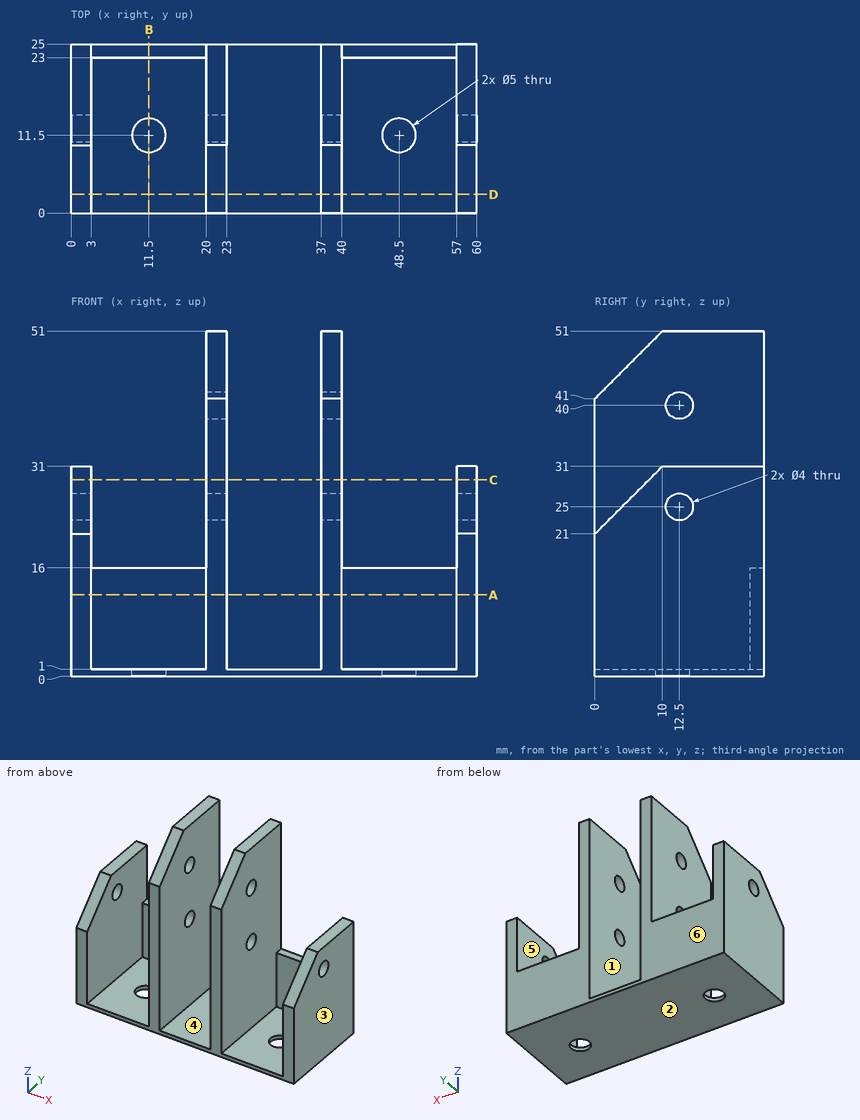
Could you check a few things on this drawing? It's one solid part, dimensions in mm from its lowest x, y, z. A direction names the side the tool comes from. Give positions to 0.01 mm unless a question says otherwise; leave off trailing zeros. Loops run counter-clockwise (first coordinate to the right, second up) from the corner with the lowest first, then second, coordinate; pieces in that order, holes last. Notation, with made-up numbers: (64, 36) -> (102, 36) arc R30 cw to (102, 59) -> close; hole circle Ø7 at (88.5, 17). An arc over 180 degrees is marked (long way). Answer as CSV lines item,"result". Start each with the question number.
(1) We'd pull the mould along X, two halves only. Please class the marked faces 1, 2 and 3: released by +X, released by -X, zero draft, split by the parting line, or undercut.
(2) If we section it at B-B on x = 11.5: Write out the boundary of the cut face in (y, z), then the cut area to 3 significant figures.
(3) Which directions (+Z, -Z, +X, -X, +Y, -Y) give clear straight access to the entire face, cutting with the end or side of a thin tool? Please do the marked faces 4, 5 and 6.
(4) I need wall thicknesses on probe 1 along X at (y, z) = (23.75, 21); probe 2 along Y at (x, z) = (38.75, 25); probe 3 along X at (y, z) = (22.25, 48). Which ranges of each line are inside material? Lowest first, please.
(5) I'm going to push flat-ended pins straight in: pin 1 Ø13.5 at (x, y) = (8, 6.5) entering from +Z; pin 2 Ø7.5 at (x, z) = (10, 5.5) entering from -Y; pin 3 Ø2 at (y, z) = (14, 35.5) entering from +X. Where does each tip first touch, or does it pass through?
(6) If we section it at C-C on z = 29: Write out the boundary of the cut face in (x, y).
(7) If we section it at D-D on y = 2.75: Write out the boundary of the cut face in (x, z).
(8) If we section it at A-A on z = 12: Write out the boundary of the cut face in (x, y), then the cut area to 3 significant figures.
Computed:
1,face 1,"undercut"
1,face 2,"zero draft"
1,face 3,"released by +X"
2,outline,"(0, 0) -> (9, 0) -> (9, 1) -> (0, 1) -> close; (14, 0) -> (25, 0) -> (25, 16) -> (23, 16) -> (23, 1) -> (14, 1) -> close"
2,area,"50.0 mm2"
3,face 4,"+Z, +Y, -Y"
3,face 5,"+Z, -Y"
3,face 6,"+Z, -Z, +X, -X, +Y"
4,probe 1,"x = 0 to 3, 20 to 23, 37 to 40, 57 to 60"
4,probe 2,"y = 0 to 10.5, 14.5 to 25"
4,probe 3,"x = 20 to 23, 37 to 40"
5,pin 1,"stops at z = 31"
5,pin 2,"stops at y = 23"
5,pin 3,"stops at x = 40"
6,outline,"(0, 8) -> (3, 8) -> (3, 25) -> (0, 25) -> close; (20, 0) -> (23, 0) -> (23, 25) -> (20, 25) -> close; (37, 0) -> (40, 0) -> (40, 25) -> (37, 25) -> close; (57, 8) -> (60, 8) -> (60, 25) -> (57, 25) -> close"
7,outline,"(0, 0) -> (60, 0) -> (60, 23.75) -> (57, 23.75) -> (57, 1) -> (40, 1) -> (40, 43.75) -> (37, 43.75) -> (37, 1) -> (23, 1) -> (23, 43.75) -> (20, 43.75) -> (20, 1) -> (3, 1) -> (3, 23.75) -> (0, 23.75) -> close"
8,outline,"(0, 0) -> (3, 0) -> (3, 23) -> (20, 23) -> (20, 0) -> (23, 0) -> (23, 25) -> (0, 25) -> close; (37, 0) -> (40, 0) -> (40, 23) -> (57, 23) -> (57, 0) -> (60, 0) -> (60, 25) -> (37, 25) -> close"
8,area,"368 mm2"
